Read the model definition and answer for the solid it produces. Units are mm, in the model's axes. Face numbers are marked on the shaded views. A direction names the side the tool comes from. Round coordinates to 2 decimals unless told otherwise and drop trailing zeros. Order: outer loops, then holes, each group sorted by start corner. A loop starts at its lowest first (then second) coordinate and runs counter-clockwise, first axis right, second up. Notation, with made-up numbers: (-39, 50) -> (-9, 50) arc R16 ccw to (-9, 70) -> close; hole circle Ø2 at (1, 48). An arc over 180 degrees is marked (long way). Answer as a JSON object with one key per item and string values. Group by question number.
Item 1: For the marked faces 4, 5, 6 and 7, determine the directions among +Z, -Z, +X, -X, +Y, -Y from which every point of the face is accessible in a straight line to the end or side of a thin tool.
Item 2: Given P1, Ø12, axis at y = -381.5, z = -28.5, coming from the +X side; P2, Ø20.5, axis at y = -328, z = -53.5, coming from the -X side; P3, Ø1.5, axis at x = 85.5, y = -282, coming from the -Z side; P4, Ø6, axis at x = -86, z = -175.5, coming from the +Y side, each flat-ended and moving along its own axis, determine where each tip first touches the part or whether it passes through.
Item 3: The mould has two halves that part along Z. Classify the marked faces 1, 2 and 3: pulls with the +Z half, pulls with the -Z half, needs draft (parallel to the pull), parting line crosses it, or undercut.
Item 4: Section B-B, the plane y = -180.5 is taken. Write down the section's boundary in (x, z), plus the area to 3 significant figures.
Item 5: Consider probe 1 along Y at (x, z) = (138, -29); probe 2 along X at (y, z) = (-344.5, -50); probe 3 along X at (y, z) = (-155, -253). Determine where each line is inside the solid, lowest interval first. Write a range as from..to.
Item 6: Section A-A, the plane x = 151 is taken. Write down the section's boundary in (y, z).
Item 7: Section C-C, the plane x = -17.5 is taken. Write down the section's boundary in (y, z), plus the area to 3 significant figures.
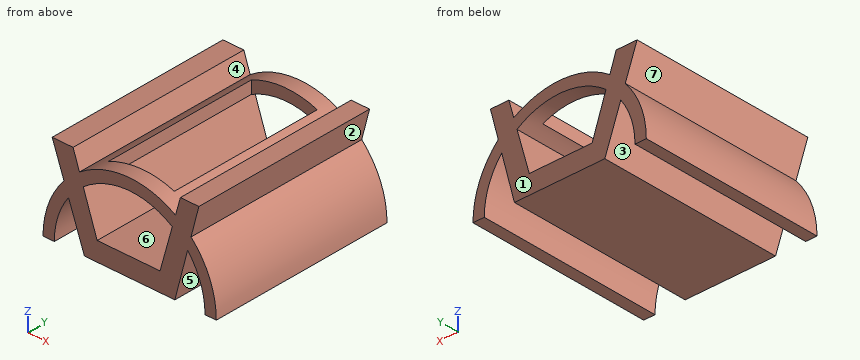
from build123d import *

# Parameters (mm, degrees)
F1_DEPTH = 624.84
F3_DEPTH = 624.84
F4_W     = 222.237472
F4_H     = 523.24
F5_DEPTH = 99.06


with BuildPart() as f1:
    # F0 (on Front) → F1 (new body)
    with BuildSketch(Plane.XZ):
        with BuildLine():
            Line((363.537534, -301.646389), (401.637534, -301.646389))
            ThreePointArc((401.637534, -301.646389), (109.905185, -8.813365), (-182.561408, -300.913066))
            Line((-182.561408, -300.913066), (-144.461408, -300.913066))
            ThreePointArc((-144.461408, -300.913066), (109.905254, -46.913399), (363.537534, -301.646389))
        make_face()
    extrude(amount=F1_DEPTH)

    # F2 (on face) → F3 (join)
    with BuildSketch(Plane.XZ.offset(624.84)):
        Polygon((-42.861408, -300.913399), (261.937534, -300.913399), (342.903882, 5.106361), (280.660063, 5.106361), (211.943924, -237.413399), (0, -237.413399), (-81.136086, 0), (-151.599751, 0), align=None)
    extrude(amount=-F3_DEPTH)

    # F4 (on face) → F5 (cut)
    with BuildSketch(Plane.XY.offset(5.106361)):
        with Locations((102.249414, -312.42)):
            Rectangle(F4_W, F4_H)
    extrude(amount=-F5_DEPTH, mode=Mode.SUBTRACT)


solid = f1.part
Values found:
{
 "1": {"face 4": "+Z, +Y, -Y", "face 5": "-Z, +Y, -Y", "face 6": "+Y, -Y", "face 7": "-X, +Y, -Y"},
 "2": {"P1": "x = 335.6", "P2": "x = -135.97", "P3": "z = -300.91", "P4": "y = 0"},
 "3": {"face 1": "needs draft", "face 2": "undercut", "face 3": "pulls with the -Z half"},
 "4": {"outline": "(-182.56, -300.91) -> (-144.46, -300.91) arc R254 cw to (-96.53, -152.41) -> (-42.86, -300.91) -> (261.94, -300.91) -> (304.89, -138.57) arc R254 cw to (363.54, -301.65) -> (401.64, -301.65) arc R292.1 ccw to (316.48, -94.76) -> (342.9, 5.11) -> (280.66, 5.11) -> (264.17, -53.1) arc R292.1 ccw to (213.37, -27.89) -> (213.37, -69.1) arc R254 cw to (253.29, -91.5) -> (211.94, -237.41) -> (0, -237.41) -> (-46.73, -100.67) arc R254 cw to (-8.87, -76.2) -> (-8.87, -33.89) arc R292.1 ccw to (-59.67, -62.81) -> (-81.14, 0) -> (-151.6, 0) -> (-111.76, -110.26) arc R292.1 ccw to start", "area": "71,100 mm2"},
 "5": {"probe 1": "-624.84..-574.04, -50.8..0", "probe 2": "-133.53..-64.05, -40.01..-8.87, 213.37..259.09, 265.05..328.32", "probe 3": "-178.61..-139.9, -60.18..274.61, 358.98..397.68"},
 "6": {"outline": "(-624.84, -300.91) -> (0, -300.91) -> (0, -237.41) -> (-624.84, -237.41) -> close; (-624.84, -50.32) -> (-574.04, -50.32) -> (-574.04, -11.77) -> (-624.84, -11.77) -> close; (-50.8, -50.32) -> (0, -50.32) -> (0, -11.77) -> (-50.8, -11.77) -> close"},
 "7": {"outline": "(-624.84, -300.91) -> (0, -300.91) -> (0, -186.21) -> (-624.84, -186.21) -> close; (-624.84, -80.96) -> (0, -80.96) -> (0, -37.89) -> (-624.84, -37.89) -> close", "area": "98,600 mm2"}
}
